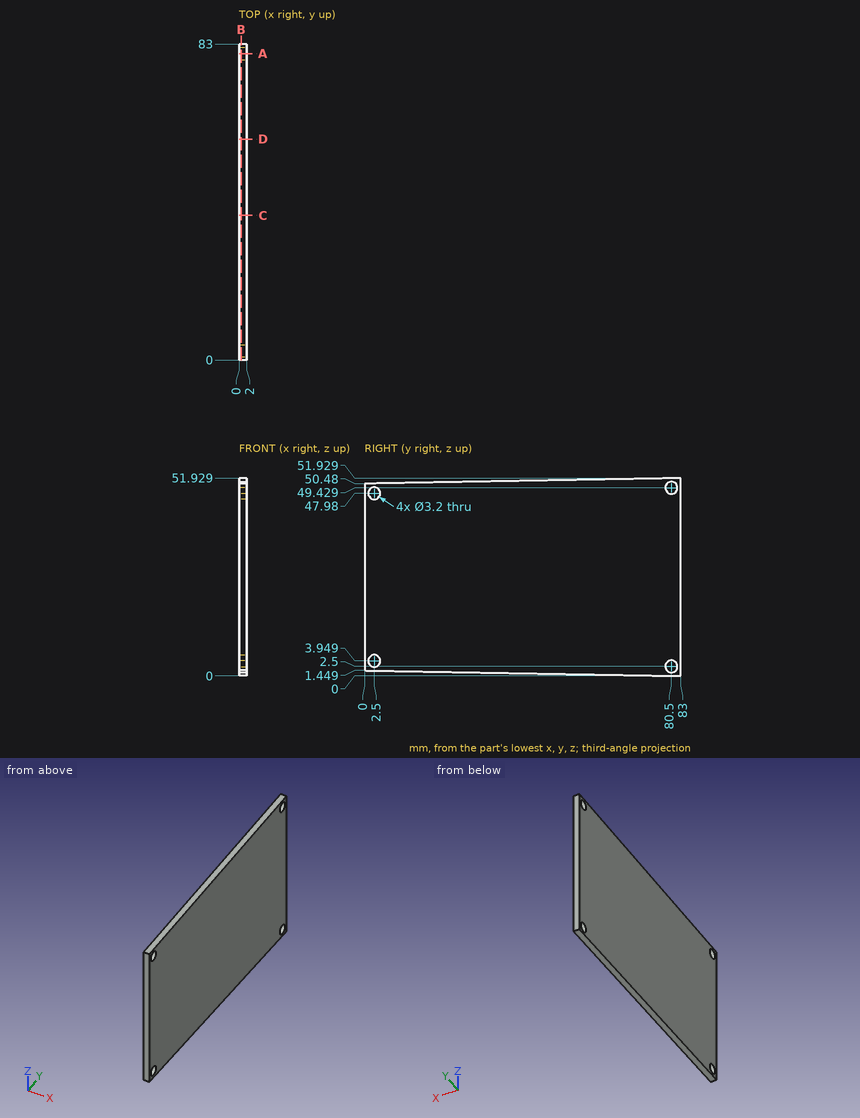
Print and shaded views of the part. All mm, measured from the part's lowest x, y and z. Round coordinates to 2 decimals unless told otherwise and drop trailing zeros. Write each loop counter-clockwise with the first axis right and the second up, starting at its lowest first coordinate (ties: lowest second). Pieces come first, ordered by that corner, then holes. Notation, with made-up numbers: (52.5, -31.5) -> (103.5, -31.5) arc R17 ccw to (103.5, -10.5) -> close; hole circle Ø9 at (61.25, 11). An arc over 180 degrees is marked (long way). Return JSON: item names as keys, results as strings. Group by question number.
Q1. Saw through at A-A on y = 80.5. Write the cut outline in (x, z) (1 decimal).
Q2. Pin check, flat tip, straight feed: pin 1 (5 mm diameter, centred on y = 80.5, z = 2.5, fed in from +X). Stop position of the tip, or through.
Q3. Probe L1, parallel to Y at x = 0.5, z = 2.5; L2, parallel to Z at x = 0.5, y = 36; L3, parallel to Z at x = 1.9, y = 9. List the from-to ranges inside material, lowest first. Write a range as [from, to].
Q4. Saw through at B-B on x = 0.55. Write the cut outline in (y, z).
Q5. Saw through at C-C on y = 38. Write the cut outline in (x, z), plus the area to 3 significant figures.
Q6. Saw through at D-D on y = 58. Write the cut outline in (x, z).
Answer:
{
 "1": {"outline": "(0, 0) -> (2, 0) -> (2, 0.9) -> (0, 0.9) -> close; (0, 4.1) -> (2, 4.1) -> (2, 47.8) -> (0, 47.8) -> close; (0, 51) -> (2, 51) -> (2, 51.9) -> (0, 51.9) -> close"},
 "2": {"pin 1": "x = 2"},
 "3": {"L1": "[0, 1.82], [3.18, 78.9], [82.1, 83]", "L2": "[0.82, 51.11]", "L3": "[1.29, 50.64]"},
 "4": {"outline": "(0, 1.45) -> (83, 0) -> (83, 51.93) -> (0, 50.48) -> close; hole circle Ø3.2 at (2.5, 3.95); hole circle Ø3.2 at (2.5, 47.98); hole circle Ø3.2 at (80.5, 2.5); hole circle Ø3.2 at (80.5, 49.43)"},
 "5": {"outline": "(0, 0.79) -> (2, 0.79) -> (2, 51.14) -> (0, 51.14) -> close", "area": "101 mm2"},
 "6": {"outline": "(0, 0.44) -> (2, 0.44) -> (2, 51.49) -> (0, 51.49) -> close"}
}
